Geometry: final body of the model. Coordinates: model frame, mm. A direction names the side the tool comes from. Coordinates: 2 decimals unless noted, no trailing zeros. Order: outer loops, then holes, each group sorted by start corner. A loop starts at its lowest first (then second) coordinate and runs counter-clockwise, first axis right, second up. Notation, with made-up numbers: M 62,48 L 71,48 A18 cw 71,70 Z; hole C -37,-25 d5. An arc over 180 degrees is marked long. Write item = value, one per line.
from build123d import *

# Parameters (mm, degrees)
CROQUIS1_W              = 42
CROQUIS1_H              = 85
CROQUIS1_R              = 2.05
SALIENTE_EXTRUIR1_DEPTH = 5
CROQUIS4_R              = 4.05
CORTAR_EXTRUIR1_DEPTH   = 2.8
CHAFL_N1_SIZE           = 4.1
CROQUIS7_R              = 5
CORTAR_EXTRUIR4_DEPTH   = 6


with BuildPart() as part:
    # Croquis1 → Saliente-Extruir1 (new body)
    with BuildSketch(Plane.XY):
        with Locations((21, 42.5)):
            Rectangle(CROQUIS1_W, CROQUIS1_H)
        with Locations((11, 76.8)):
            Circle(CROQUIS1_R, mode=Mode.SUBTRACT)
        with Locations((31, 76.8)):
            Circle(CROQUIS1_R, mode=Mode.SUBTRACT)
        with Locations((31, 56.8)):
            Circle(CROQUIS1_R, mode=Mode.SUBTRACT)
        with Locations((11, 56.8)):
            Circle(CROQUIS1_R, mode=Mode.SUBTRACT)
    extrude(amount=SALIENTE_EXTRUIR1_DEPTH)

    # Croquis4 → Cortar-Extruir1 (cut)
    with BuildSketch(Plane.XY.offset(5)):
        with Locations((11, 76.8)):
            Circle(CROQUIS4_R)
        with Locations((11, 56.8)):
            Circle(CROQUIS4_R)
        with Locations((31, 56.8)):
            Circle(CROQUIS4_R)
        with Locations((31, 76.8)):
            Circle(CROQUIS4_R)
    extrude(amount=-CORTAR_EXTRUIR1_DEPTH, mode=Mode.SUBTRACT)

    # Chaflán1
    chafl_n1_edges = [part.edges().sort_by_distance(p)[0] for p in [
        (42, 0, 2.5),
        (0, 0, 2.5),
    ]]
    chamfer(chafl_n1_edges, length=CHAFL_N1_SIZE)

    # Croquis7 → Cortar-Extruir4 (cut, through all)
    with BuildSketch(Plane.XY.offset(5)):
        with Locations((21, 21.08)):
            Circle(CROQUIS7_R)
    extrude(amount=-CORTAR_EXTRUIR4_DEPTH, mode=Mode.SUBTRACT)


solid = part.part
1) Set-up query: faces 1 (the face through (10.122, 52.846, 3.62)), 2 (the face through (30.733, 78.833, 1.085)). Return all of +Z, -Z, +X, -X, +Y, -Y with unobstructed straight access to the full face (end or side cutting, diameter ignored); none if empty.
Numbers:
face_1 = +Z
face_2 = +Z, -Z
2) Section A-A, the plane x = 11. Return loops of the section in (y, z), and give its area (3 significant figures).
Numbers:
outline = M 0,0 L 54.75,0 L 54.75,2.2 L 52.75,2.2 L 52.75,5 L 0,5 Z; M 58.85,0 L 74.75,0 L 74.75,2.2 L 72.75,2.2 L 72.75,5 L 60.85,5 L 60.85,2.2 L 58.85,2.2 Z; M 78.85,0 L 85,0 L 85,5 L 80.85,5 L 80.85,2.2 L 78.85,2.2 Z
area = 362 mm²
3) Pin query (flat end, axial travel): pin 1 (5.5 mm diameter, centred on x = 11, y = 76.8, fed in from -Z); pin 2 (2.5 mm diameter, centred on x = 32, y = 58, fed in from +Z). Return the tip coordinate at first contact, or that it passes through.
Numbers:
pin_1 = 0
pin_2 = 2.2
4) Section D-D, the plane z = 0.8. Return loops of the section in (x, y), and give its area (3 significant figures).
Numbers:
outline = M 0,4.1 L 4.1,0 L 37.9,0 L 42,4.1 L 42,85 L 0,85 Z; hole C 11,56.8 d4.1; hole C 11,76.8 d4.1; hole C 21,21.08 d10; hole C 31,56.8 d4.1; hole C 31,76.8 d4.1
area = 3,420 mm²
5) Line query: L1, parallel to Y at x = 11, z = 3.05; L2, parallel to X at y = 76.8, z = 1; L3, parallel to Y at x = 31, z = 1.75. Output: solid intervals per line, ascending.
Numbers:
L1 = 0 to 52.75, 60.85 to 72.75, 80.85 to 85
L2 = 0 to 8.95, 13.05 to 28.95, 33.05 to 42
L3 = 0 to 54.75, 58.85 to 74.75, 78.85 to 85
6) Mould query, pull axis Y, two halves, no side actions, for faces 3 (the face through (21, 0, 2)), 4 (the face through (30, 79, 2.2)), 5 (the face through (0, 44, 2)), 6 (the face through (21, 85, 2)). Classes: pulls with the +Y half, pulls with the -Y half, needs draft (parallel to the pull), parting line crosses it, or undercut.
Numbers:
face_3 = pulls with the -Y half
face_4 = undercut
face_5 = needs draft
face_6 = pulls with the +Y half
7) Section B-B, the plane y = 56.8. Return loops of the section in (x, z), and give its area (3 significant figures).
Numbers:
outline = M 0,0 L 8.95,0 L 8.95,2.2 L 6.95,2.2 L 6.95,5 L 0,5 Z; M 13.05,0 L 28.95,0 L 28.95,2.2 L 26.95,2.2 L 26.95,5 L 15.05,5 L 15.05,2.2 L 13.05,2.2 Z; M 33.05,0 L 42,0 L 42,5 L 35.05,5 L 35.05,2.2 L 33.05,2.2 Z
area = 147 mm²
8) Section C-C, the plane x = 18. Return loops of the section in (y, z).
Numbers:
outline = M 0,0 L 17.08,0 L 17.08,5 L 0,5 Z; M 25.08,0 L 85,0 L 85,5 L 25.08,5 Z
